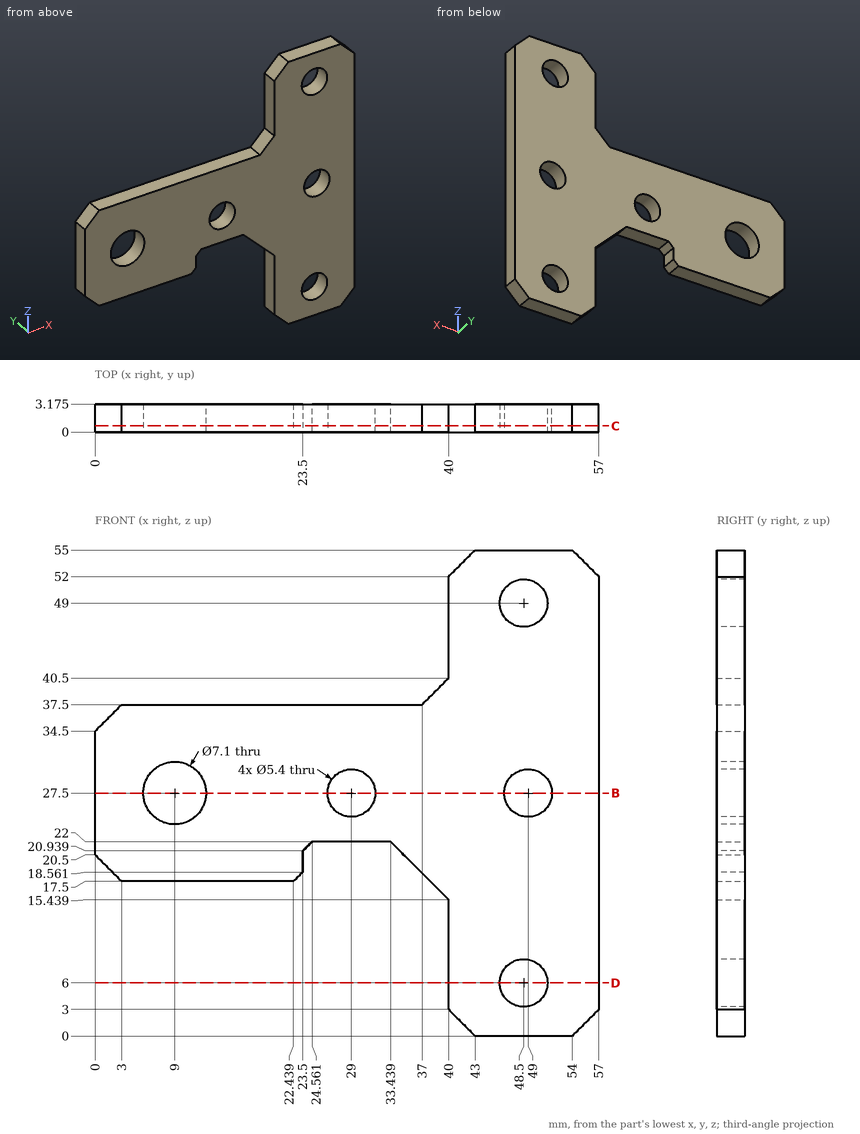
Here's the drawing with two shaded views (mm, measured from the low corner). I have some questions. Coordinates: 2 decimals unless noted, no trailing zeros. Write each loop counter-clockwise with the first axis right and the second up, starting at its lowest first coordinate (ties: lowest second). Pieces come first, ordered by that corner, then holes.
Item 1: I want a section at C-C on y = 0.7. Write out the boundary of the cut face in (x, z), and give its area (3 significant figures).
Item 2: I want a section at D-D on z = 6. Write out the boundary of the cut face in (x, y) (1 decimal).
Item 3: Will these pins go through, and if not, where does the flat tip stop? pin 1 (5 mm diameter, centred on x = 48.5, z = 49, fed in from -Y); pin 2 (11.5 mm diameter, centred on x = 9, z = 27.5, fed in from -Y); pin 3 (1.6 mm diameter, centred on x = 28.5, y = 1, fed in from -Z).
Item 4: I want a section at B-B on z = 27.5. Count the separate pieces of the cut face and the enclosed holes in it, and give its area (3 significant figures).
Item 5: If I drill on line 1 (X direction, y = 2.5, z = 27.5); line 2 (Z direction, x = 9, y = 1.8); line 3 (X direction, y = 0.7, z = 49), over which ranges is the centre line in solid material (lowest first)?
Findings below:
1. outline: (0, 20.5) - (3, 17.5) - (22.44, 17.5) - (23.5, 18.56) - (23.5, 20.94) - (24.56, 22) - (33.44, 22) - (40, 15.44) - (40, 3) - (43, 0) - (54, 0) - (57, 3) - (57, 52) - (54, 55) - (43, 55) - (40, 52) - (40, 40.5) - (37, 37.5) - (3, 37.5) - (0, 34.5) - close; hole circle Ø7.1 at (9, 27.5); hole circle Ø5.4 at (29, 27.5); hole circle Ø5.4 at (48.5, 6); hole circle Ø5.4 at (48.5, 49); hole circle Ø5.4 at (49, 27.5)
1. area: 1,530 mm2
2. outline: (40, 0) - (45.8, 0) - (45.8, 3.2) - (40, 3.2) - close; (51.2, 0) - (57, 0) - (57, 3.2) - (51.2, 3.2) - close
3. pin 1: passes through
3. pin 2: stops at y = 0
3. pin 3: stops at z = 22
4. separate pieces: 4
4. enclosed holes: 0
4. area: 124 mm2
5. line 1: x = 0 to 5.45, 12.55 to 26.3, 31.7 to 46.3, 51.7 to 57
5. line 2: z = 17.5 to 23.95, 31.05 to 37.5
5. line 3: x = 40 to 45.8, 51.2 to 57
